```python
from build123d import *

# Parameters (mm, degrees)
SKETCH_1_W      = 80
SKETCH_1_H      = 42
SKETCH_1_R      = 1.6
EXTRUDE_1_DEPTH = 3
FILLET_1_R      = 2
FILLET_2_R      = 2


with BuildPart() as part:
    # 草图1 → 凸台-拉伸1 (new body)
    with BuildSketch(Plane(origin=(0, 0, 0), x_dir=(1, 0, 0), z_dir=(0, 1, 0))):
        Rectangle(SKETCH_1_W, SKETCH_1_H)
        with Locations(Location((-37, -18, 0), (0, 0, 270))):
            Circle(SKETCH_1_R, mode=Mode.SUBTRACT)
        Polygon((34, -15), (4, -15), (4, -10), (10, -10), (10, -4), (34, -4), align=None, mode=Mode.SUBTRACT)
        Polygon((-10, -10), (-4, -10), (-4, -15), (-34, -15), (-34, -4), (-10, -4), align=None, mode=Mode.SUBTRACT)
        Polygon((-34, 4), (-34, 15), (-4, 15), (-4, 10), (-10, 10), (-10, 4), align=None, mode=Mode.SUBTRACT)
        Polygon((4, 15), (34, 15), (34, 4), (10, 4), (10, 10), (4, 10), align=None, mode=Mode.SUBTRACT)
        with Locations(Location((37, -18, 0), (0, 0, 270))):
            Circle(SKETCH_1_R, mode=Mode.SUBTRACT)
        with Locations(Location((-37, 18, 0), (0, 0, 270))):
            Circle(SKETCH_1_R, mode=Mode.SUBTRACT)
        with Locations(Location((37, 18, 0), (0, 0, 270))):
            Circle(SKETCH_1_R, mode=Mode.SUBTRACT)
    extrude(amount=EXTRUDE_1_DEPTH)

    # 圆角1
    fillet_1_edges = [part.edges().sort_by_distance(p)[0] for p in [
        (34, 1.5, 15),
        (34, 1.5, 4),
        (10, 1.5, 4),
        (10, 1.5, 10),
        (4, 1.5, 10),
        (4, 1.5, 15),
        (-4, 1.5, 10),
        (-10, 1.5, 10),
        (-10, 1.5, 4),
        (-34, 1.5, 4),
        (-34, 1.5, 15),
        (-4, 1.5, 15),
        (-4, 1.5, -15),
        (-34, 1.5, -15),
        (-34, 1.5, -4),
        (-10, 1.5, -4),
        (-10, 1.5, -10),
        (-4, 1.5, -10),
        (34, 1.5, -4),
        (34, 1.5, -15),
        (4, 1.5, -15),
        (4, 1.5, -10),
        (10, 1.5, -10),
        (10, 1.5, -4),
    ]]
    fillet(fillet_1_edges, radius=FILLET_1_R)

    # 圆角2
    fillet_2_edges = [part.edges().sort_by_distance(p)[0] for p in [
        (-40, 1.5, -21),
        (40, 1.5, -21),
        (40, 1.5, 21),
        (-40, 1.5, 21),
    ]]
    fillet(fillet_2_edges, radius=FILLET_2_R)


solid = part.part
```
Geometry check sheet. Reference: the model listing, model coordinates, mm. A direction names the side the tool comes from. Round coordinates to 2 decimals unless told otherwise and drop trailing zeros. Order: outer loops, then holes, each group sorted by start corner. A loop starts at its lowest first (then second) coordinate and runs counter-clockwise, first axis right, second up. Notation, with made-up numbers: M 84,-34.5 L 109,-34.5 A20 cw 109,-0.5 Z; hole C -32.5,-9 d9. An arc over 180 degrees is marked long. Answer as CSV lines item,"result".
1) Sectioned sample at A-A on z = 18. Record the cut outline in (x, y).
Entries:
outline,"M -40,0 L -38.6,0 L -38.6,3 L -40,3 Z; M -35.4,0 L 35.4,0 L 35.4,3 L -35.4,3 Z; M 38.6,0 L 40,0 L 40,3 L 38.6,3 Z"
2) Thickness scan on probe 1 along X at (y, z) = (2.15, -6.5); probe 2 along X at (y, z) = (1.4, 18); probe 3 along Z at (x, y) = (12.5, 0.5). Record the ranges inside material, lowest first. Write a range as [from, to].
Entries:
probe 1,"[-40, -34], [-10, 10], [34, 40]"
probe 2,"[-40, -38.6], [-35.4, 35.4], [38.6, 40]"
probe 3,"[-21, -15], [-4, 4], [15, 21]"
3) Mould release check, pull along Z, two halves, no side actions. Record for faces 1 (the face through (-34, 1, 10)), 2 (the face through (39.4, 1.52, 20.43)), 3 (the face through (33.43, 1.52, 14.4)): +Z half, -Z half, draft (parallel to the pull), parting line (faces both ways), or undercut.
Entries:
face 1,"undercut"
face 2,"+Z half"
face 3,"undercut"
4) Tool access check on faces 4 (the face through (-4.6, 1.52, -14.43)), 5 (the face through (-1, 1, 21)). Record the directions out of +Z, -Z, +X, -X, +Y, -Y that give a thin tool (end or side, any length) a straight path to the whole face; none if there is none.
Entries:
face 4,"+Y, -Y"
face 5,"+Z, +X, -X, +Y, -Y"
5) Sectioned sample at B-B on x = 37. Record the cut outline in (y, z), and give its area (3 significant figures).
Entries:
outline,"M 0,-21 L 3,-21 L 3,-19.6 L 0,-19.6 Z; M 0,-16.4 L 3,-16.4 L 3,16.4 L 0,16.4 Z; M 0,19.6 L 3,19.6 L 3,21 L 0,21 Z"
area,"107 mm2"
